For this review, take the finished solid that the model builds, in its own axes (mm). A direction names the side the tool comes from. Round coordinates to 2 decimals unless told otherwise and drop trailing zeros. Order: outer loops, then holes, each group sorted by start corner. A loop starts at its lowest first (then second) coordinate and runs counter-clockwise, first axis right, second up. Notation, with made-up numbers: (80.5, 29) - (88.5, 29) arc R15 cw to (88.5, 46) - close; hole circle Ø5 at (64, 57.5). An arc over 180 degrees is marked (long way). Write each question's results on one line, items separated by ' | '. Start each with the question number.
(1) For L1, parallel to X at y = 25, z = 39.5; L2, parallel to Z at x = 9, y = -15.5, list the stretches that pass through material, from the lowest coordinate up. Write a range as from..to.
(2) For faces 1 (the flat face through (-13, 50.8, -14)), 2 (the flat face through (-1.43, -1, 21)), list the 3-axis set-ups (+Z, -Z, +X, -X, +Y, -Y) from which the entire face can be reached by the end or side of a thin tool; tool diameter is ignored.
(3) Insertion check: pin 1 Ø5 at (x, y) = (10, 26) entering from +Z. The pin has a flat end and moves straight along its axis. Give the tip position at first contact, or say it passes through.
(4) Take a section at A-A, the plane y = -30. Give the boundary of the cut face in (x, z), plus the area to 3 significant figures.
(5) Take a section at B-B, the plane z = 23.5. Give the boundary of the cut face in (x, y).
(6) Take a section at C-C, the plane x = 34.5. Give the boundary of the cut face in (y, z).
```python
from build123d import *

# Parameters (mm, degrees)
F0_W     = 50.8
F0_H     = 50.8
F1_DEPTH = 50.8


with BuildPart() as f1:
    # F0 (on Front) → F1 (new body, symmetric)
    with BuildSketch(Plane.XZ):
        Polygon((-52.229806, 47.116514), (-52.229806, -54.483486), (-1.429806, -54.483486), (-1.429806, -3.683486), (-1.429806, 47.116514), align=None)
        with Locations((23.970194, -29.083486)):
            Rectangle(F0_W, F0_H)
    extrude(amount=F1_DEPTH, both=True)


solid = f1.part
```
Results below:
1) L1: x = -52.23..-1.43 | L2: z = -54.48..-3.68
2) face 1: +Z, -Z, +X, -X, +Y | face 2: +Z, +X, +Y, -Y
3) pin 1: stops at z = -3.68
4) outline: (-52.23, -54.48) - (49.37, -54.48) - (49.37, -3.68) - (-1.43, -3.68) - (-1.43, 47.12) - (-52.23, 47.12) - close | area: 7,740 mm^2
5) outline: (-52.23, -50.8) - (-1.43, -50.8) - (-1.43, 50.8) - (-52.23, 50.8) - close
6) outline: (-50.8, -54.48) - (50.8, -54.48) - (50.8, -3.68) - (-50.8, -3.68) - close
